The model under review builds one solid part; all positions refer to its coordinate system, in mm. Face numbers are marked on the shaded views. A direction names the side the tool comes from. Coordinates: 2 decimals unless noted, no trailing zeros. Order: outer loops, then holes, each group sorted by start corner. A loop starts at its lowest first (then second) coordinate and runs counter-clockwise, first axis right, second up. Notation, with made-up numbers: M -15,3 L 8,3 A23 cw 8,13 Z; hole C 35,-2.5 d5. An arc over 180 degrees is marked long. Answer in a Markdown table with one row per item.
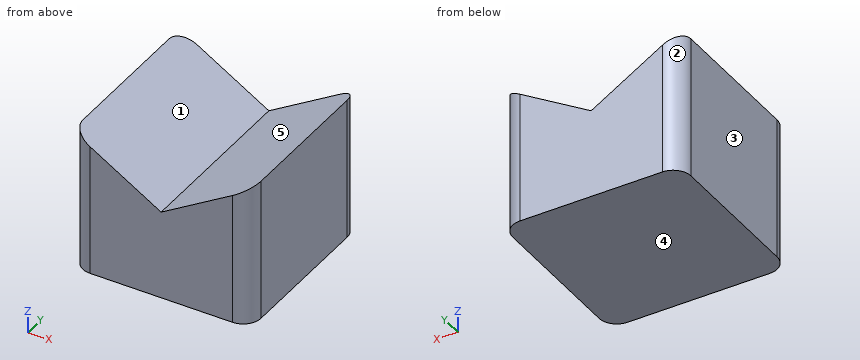
from build123d import *

# Parameters (mm, degrees)
F1_DEPTH = 20.32
F4_DEPTH = 25.4


with BuildPart() as f1:
    # F0 (on Top) → F1 (new body)
    with BuildSketch(Plane.XY):
        with BuildLine():
            Line((22.86, 0), (2.54, 0))
            ThreePointArc((2.54, 0), (0.7439487758, -0.7439487758), (0, -2.54))
            Line((0, -2.54), (0, -22.86))
            ThreePointArc((0, -22.86), (0.7439487758, -24.6560512242), (2.54, -25.4))
            Line((2.54, -25.4), (22.86, -25.4))
            ThreePointArc((22.86, -25.4), (24.6560512242, -24.6560512242), (25.4, -22.86))
            Line((25.4, -22.86), (25.4, -2.54))
            ThreePointArc((25.4, -2.54), (24.6560512242, -0.7439487758), (22.86, 0))
        make_face()
    extrude(amount=F1_DEPTH)

    # F2 (on face) → F4 (cut)
    with BuildSketch(Plane.XZ.offset(25.4)):
        Polygon((2.54, 18.796), (12.7, 12.7), (22.86, 18.796), (22.86, 20.32), (2.54, 20.32), align=None)
        Polygon((0, 20.32), (2.54, 18.796), (2.54, 20.32), align=None)
        Polygon((22.86, 20.32), (22.86, 18.796), (25.4, 20.32), align=None)
    extrude(amount=-F4_DEPTH, mode=Mode.SUBTRACT)


solid = f1.part
(1) The part is to be moulded in two halves that separate along X. For the marked faces 3, 4 and 5, say which applies: +X half, -X half, draft (parallel to the pull), parting line (faces both ways), or undercut.
Report:
| item | result |
|---|---|
| face 3 | -X half |
| face 4 | draft |
| face 5 | undercut |
(2) Take a section at A-A (z = 18.25). Write out the cut boundary in (x, y), then the cut area to 3 significant figures.
Report:
| item | result |
|---|---|
| outline | M 0,-22.86 A2.54 ccw 2.54,-25.4 L 3.45,-25.4 L 3.45,0 L 2.54,0 A2.54 ccw 0,-2.54 Z; M 21.95,-25.4 L 22.86,-25.4 A2.54 ccw 25.4,-22.86 L 25.4,-2.54 A2.54 ccw 22.86,0 L 21.95,0 Z |
| area | 170 mm^2 |
(3) Take a section at D-D (x = 17.25). Write out the cut boundary in (y, z).
Report:
| item | result |
|---|---|
| outline | M -25.4,0 L 0,0 L 0,15.43 L -25.4,15.43 Z |
(4) Machinability: for the marked faces 1 and 2, which of the approach directions +Z, -Z, +X, -X, +Y, -Y give a long, thin tool a straight path to every point of the face, cutting with its end or side? Answer none if there is none.
Report:
| item | result |
|---|---|
| face 1 | +Z, +Y, -Y |
| face 2 | +Z, -Z, -X, +Y |
(5) To check wall thickness, follow line 1 (X direction, y = -12.75, z = 17.5); line 2 (X direction, y = -20.75, z = 17.75); line 3 (Y direction, x = 23, z = 4.25). State the ranges of each line that lie inside material, in increasing order. Write a range as [from, to].
Report:
| item | result |
|---|---|
| line 1 | [0, 4.7], [20.7, 25.4] |
| line 2 | [0, 4.28], [21.12, 25.4] |
| line 3 | [-25.4, 0] |
(6) Insertion check: P1, Ø12, axis at x = 7, y = -17, coming from the +Z side; P2, Ø1, axis at x = 4.5, y = -17, coming from the +Z side. Each pin has a flat end and moves straight along its axis. Give the tip position at first contact, or say it passes through.
Report:
| item | result |
|---|---|
| P1 | z = 19.72 |
| P2 | z = 17.92 |
(7) Take a section at C-C (x = 7). Write out the cut boundary in (y, z).
Report:
| item | result |
|---|---|
| outline | M -25.4,0 L 0,0 L 0,16.12 L -25.4,16.12 Z |
(8) Take a section at B-B (y = -17.75). Write out the cut boundary in (x, z), then the cut area to 3 significant figures.
Report:
| item | result |
|---|---|
| outline | M 0,0 L 25.4,0 L 25.4,20.32 L 12.7,12.7 L 0,20.32 Z |
| area | 419 mm^2 |
